Here's how the part is built. I have some questions about the finished solid (model axes, mm). Round coordinates to 2 decimals unless told otherwise and drop trailing zeros. Loops run counter-clockwise (first coordinate to the right, second up) from the corner with the lowest first, then second, coordinate; pieces in that order, holes last. Notation, with made-up numbers: M 21.25,48.25 L 73.25,48.25 A26 ccw 73.25,71.25 Z; hole C -0.75,88 d2. An arc over 180 degrees is marked long. Answer as a JSON object with one key per item and string values.
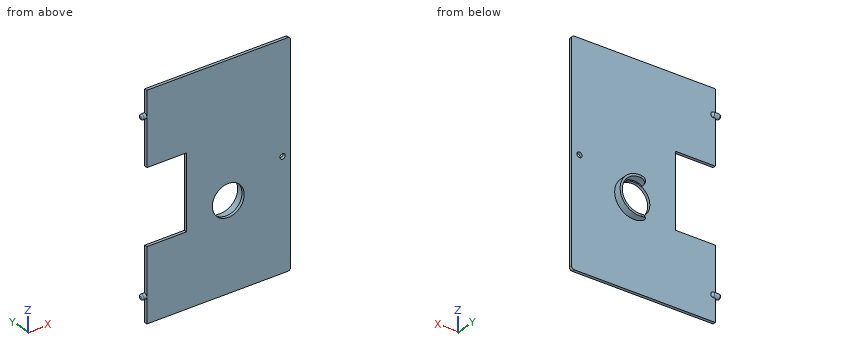
Autodesk Inventor part; units mm, degrees
ref_plane "YZ Plane" through (0, 0, 0) normal (1, 0, 0) x (0, 1, 0)
ref_plane "XZ Plane" through (0, 0, 0) normal (0, 1, 0) x (-1, 0, 0)
ref_plane "XY Plane" through (0, 0, 0) normal (0, 0, 1) x (1, 0, 0)
sketch "Sketch1" plane through (0, 0, 0) normal (0, 1, 0) x (-1, 0, 0)
  line L0 (-48.571, 73.95) -> (48.571, 73.95)
  line L1 (48.571, 73.95) -> (48.571, -73.95)
  line L2 (48.571, -73.95) -> (-48.571, -73.95)
  line L3 (-48.571, -73.95) -> (-48.571, 73.95)
  line L4 (-48.571, 73.95) -> (48.571, -73.95) construction
  line L5 (48.571, 73.95) -> (-48.571, -73.95) construction
  circle A0 centre (-43.171, 0) radius 1.75
  line L6 (-48.571, -73.95) -> (-48.571, -59.45)
  circle A1 centre (-6.429, -15) radius 10.75
  line L7 (-67.9994, 0) -> (67.9994, 0) construction
  point P0 (0, 0)
  dimension "d0" = 97.142
  dimension "d1" = 147.9
  dimension "d3" = 3.5
  dimension "d54" = 55
  dimension "d61" = 5.4
  dimension "d62" = 15
  dimension "d63" = 21.5
extrude "Lid Shape" add sketch "Sketch1" along normal blind 2
sketch "Sketch2" plane through (0, 2, 0) normal (0, 1, 0) x (1, 0, 0)
  circle A0 centre (6.429, 15) radius 10.75
  circle A1 centre (6.429, 15) radius 11.5
  circle A2 centre (6.429, 15) radius 13
  line L0 (6.429, 15) -> (-0.071, 3.7417)
  line L1 (6.429, 15) -> (19.429, 15) construction
  line L2 (6.429, 15) -> (-0.071, 26.2583)
  circle A3 centre (6.429, 15) radius 10.75 construction
  point P0 (0.679, 24.9593)
  point P1 (0.679, 5.0407)
  dimension "d64" = 26
  dimension "d65" = 23
  dimension "d66" = 120
  dimension "d67" = 120
extrude "Switch Protector" add sketch "Sketch2" along normal blind 5 contours L2 A2 L0 A1 picked at (18.7089, 13.1166)
fillet "Fillet1" radius 5 2 edges at (0.304, 7, -4.3912) (0.304, 7, -25.6088)
fillet "Fillet2" radius 2 2 edges at (48.571, 1, 73.95) (48.571, 1, -73.95)
sketch "Sketch4" plane through (-48.571, 0, -73.95) normal (-1, 0, 0) x (0, 0, 1)
  line L0 (16.95, 0) -> (16.95, 1.75) construction
  circle A0 centre (16.95, 1.75) radius 1.75
  circle A1 centre (73.95, 1.75) radius 1.75
  circle A2 centre (130.95, 1.75) radius 1.75
  line L1 (0, 2) -> (147.9, 2)
  line L2 (0, 0) -> (147.9, 0)
  line L3 (147.9, 0) -> (147.9, 2)
  line L4 (0, 2) -> (147.9, 2)
  line L5 (0, 0) -> (0, 2)
  line L6 (73.95, 4.2) -> (73.95, -0.7) construction
  point P0 (73.95, 0)
  dimension "d68" = 3.5
  dimension "d69" = 57
  dimension "d70" = 57
extrude "Peg Connectors" add sketch "Sketch4" along normal blind 3 and the other way blind 3 contours A0 L1 | L1 A0 | L1 A1 | A1 L1 | A2 L1 | A2 L1
fillet "Fillet5" radius 1.5 3 edges at (-45.571, 3.5, 57) (-45.571, 3.5, 0) (-45.571, 3.5, -57)
fillet "Fillet6" radius 1 3 edges at (-51.571, 1.75, 55.25) (-51.571, 1.75, -1.75) (-51.571, 1.75, -58.75)
sketch "Sketch7" plane through (0, 2, 0) normal (0, 1, 0) x (1, 0, 0)
  line L0 (-21.771, -25) -> (-21.771, 25)
  line L1 (-21.771, 25) -> (-55.771, 25)
  line L2 (-55.771, 25) -> (-55.771, -25)
  line L3 (-55.771, -25) -> (-21.771, -25)
  line L4 (-48.571, -1.7321) -> (-48.571, -55.2679) construction
  line L5 (-76.6394, 0) -> (69.4394, 0) construction
  point P0 (0, 0)
  dimension "d60" = 50
  dimension "d71" = 34
  dimension "d72" = 26.8
extrude "Weapon Hole" cut sketch "Sketch7" along normal mid plane 6.7625
properties part number "Base Shell Top V3"
Item 1: For P1, Ø1, axis at y = 1.5, z = 9.5, coming from the -X side; P2, Ø10, axis at x = -27, z = 34, coming from the -Y side; P3, Ø0.6, axis at y = 1, z = 37.5, coming from the -X side; P4, Ø2, axis at y = 3.5, z = -37, coming from the +X side, each with a flat end and sliding along its axis, tell me the tip position at first contact or that it passes through.
Solution:
{"P1": "stops at x = -21.77", "P2": "stops at y = 0", "P3": "stops at x = -48.57", "P4": "passes through"}
Item 2: I want a section at D-D on x = -18.5. List the corners of the cut face in (y, z) for me.
Solution:
{"outline": "M 0,-73.95 L 2,-73.95 L 2,73.95 L 0,73.95 Z"}
Item 3: I want a section at A-A on x = -35.5. List the corners of the cut face in (y, z) for me.
Solution:
{"outline": "M 0,-73.95 L 2,-73.95 L 2,-25 L 0,-25 Z; M 0,25 L 2,25 L 2,73.95 L 0,73.95 Z"}
Item 4: I want a section at B-B on z = -15. List the corners of the cut face in (x, y) for me.
Solution:
{"outline": "M -21.77,0 L -4.32,0 L -4.32,2 L -21.77,2 Z; M 17.18,0 L 48.57,0 L 48.57,2 L 19.43,2 L 19.43,7 L 17.93,7 L 17.93,2 L 17.18,2 Z"}
Item 5: If I drill on L1, parallel to Z at x = -42, y = 1.25; L2, parallel to X at y = 4.1, z = -15; L3, parallel to X at y = 0.5, z = -51, over which ranges is the centre line in solid material (lowest first)? Write a range as from..to.
Solution:
{"L1": "z = -73.95..-25, 25..73.95", "L2": "x = 17.93..19.43", "L3": "x = -48.57..48.57"}
Item 6: I want a section at C-C on z = 0. List the corners of the cut face in (x, y) for me, plus the area to 3 significant figures.
Solution:
{"outline": "M -21.77,0 L 41.42,0 L 41.42,2 L -21.77,2 Z; M 44.92,0 L 48.57,0 L 48.57,2 L 44.92,2 Z", "area": "134 mm2"}
